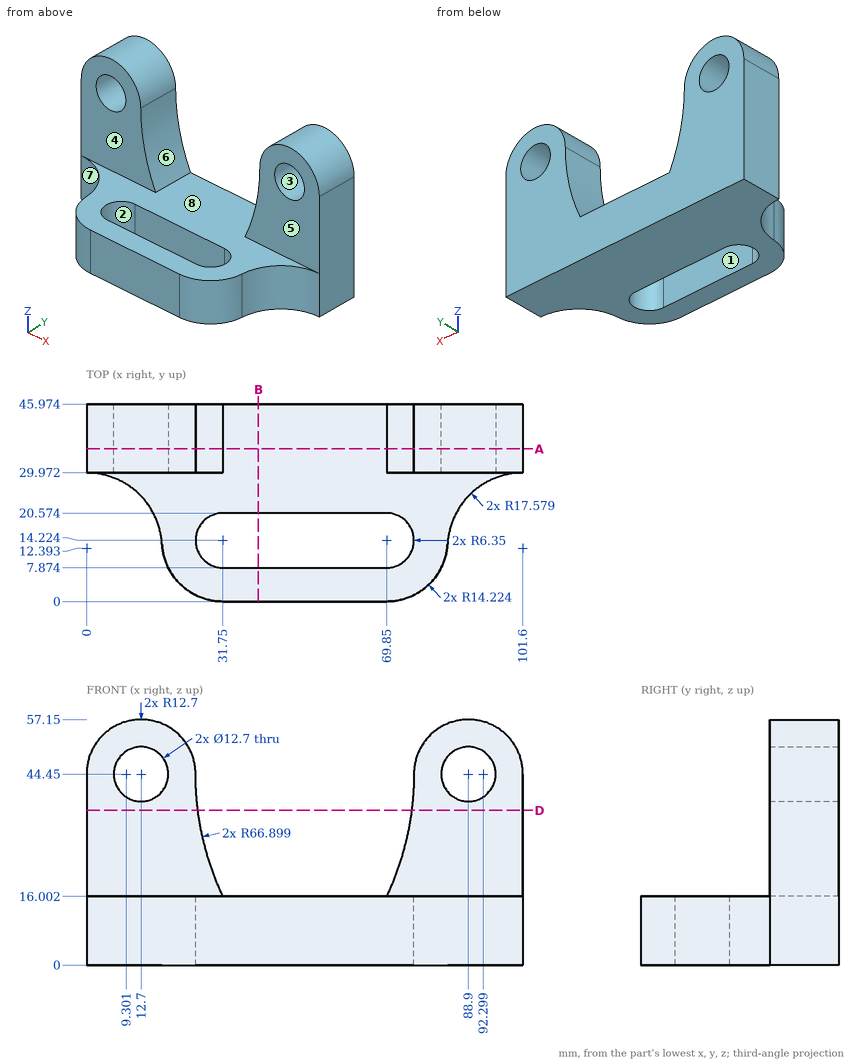
Answer from the drawing. Dimensions are ordinates in mm from the lowest x, y and z of the part. A direction names the side the tool comes from. Round coordinates to 2 decimals unless told otherwise and drop trailing zeros. Write each loop counter-clockwise with the first axis right and the second up, starting at its lowest first coordinate (ties: lowest second). Pieces come first, ordered by that corner, then holes. Notation, with made-up numbers: M 35,44 L 91,44 A29 ccw 91,80 Z; hole C 59,23.5 d10. An arc over 180 degrees is marked long. Write each question's results on one line, items separated by ' | '. Start each with the question number.
Item 1: Which of the six approach directions +Z, -Z, +X, -X, +Y, -Y give full straight-line access (tool end or side, diameter ignored) to the marked faces 5, 6, 7 and 8?
Item 2: The mould has two halves that part along Y. Classify the marked faces 1, 2, 3 and 4: +Y half, -Y half, draft (parallel to the pull), parting line (faces both ways), or undercut.
Item 3: Find section B-B on x = 40. Write down the section's boundary in (y, z).
Item 4: Straight lines are drawn through the part: probe 1 along Z at (x, y) = (12.7, 39.5); probe 2 along X at (y, z) = (42, 40); probe 3 along Z at (x, y) = (67.5, 6). For each, find the intervals that lie inside material, in ascending order.
Item 5: Find section D-D on z = 36. Write down the section's boundary in (x, y) (1 decimal), and give its area (3 significant figures).
Item 6: Find section A-A on y = 35.5. Write down the section's boundary in (x, z).
Item 7: Given pin 1 Ø4 at (x, y) = (18, 16.5) entering from +Z; pin 2 Ø16 at (x, z) = (22, 41) entering from -Y, each flat-ended and moving along its own axis, determine where each tip first touches the part or whether it passes through.
Answer block:
1) face 5: +Z, +X, -X, -Y | face 6: +Z, +Y, -Y | face 7: +Z, -Z, -X, -Y | face 8: +Z, -Y
2) face 1: undercut | face 2: undercut | face 3: draft | face 4: -Y half
3) outline: M 0,0 L 7.87,0 L 7.87,16 L 0,16 Z; M 20.57,0 L 45.97,0 L 45.97,16 L 20.57,16 Z
4) probe 1: z = 0 to 38.1, 50.8 to 57.15 | probe 2: x = 0 to 8.17, 17.23 to 25.55, 76.05 to 84.37, 93.43 to 101.6 | probe 3: z = 0 to 16
5) outline: M 0,30 L 25.9,30 L 25.9,46 L 0,46 Z; M 75.7,30 L 101.6,30 L 101.6,46 L 75.7,46 Z | area: 830 mm²
6) outline: M 0,0 L 101.6,0 L 101.6,44.45 A12.7 ccw 76.2,44.45 A66.9 cw 69.85,16 L 31.75,16 A66.9 cw 25.4,44.45 A12.7 ccw 0,44.45 Z; hole C 12.7,44.45 d12.7; hole C 88.9,44.45 d12.7
7) pin 1: stops at z = 16 | pin 2: stops at y = 29.97
